from build123d import *

# Parameters (mm, degrees)
SKETCH1_R             = 8
BOSS_EXTRUDE1_DEPTH   = 47.5
BOSS_EXTRUDE2_START   = 15
BOSS_EXTRUDE2_DEPTH   = 10
SKETCH3_R             = 9
BOSS_EXTRUDE3_DEPTH   = 4
LPATTERN1_COUNT       = 6
LPATTERN1_PITCH       = 95
BODY_MOVE_COPY1_ANGLE = 60
BODY_MOVE_COPY2_ANGLE = 120
BODY_MOVE_COPY3_ANGLE = 60
BODY_MOVE_COPY4_ANGLE = 120
BODY_MOVE_COPY5_ANGLE = 180
BOSS_EXTRUDE4_START   = 10
SKETCH4_R             = 8
BOSS_EXTRUDE4_DEPTH   = 10
BOSS_EXTRUDE5_START   = 5
SKETCH5_R             = 9
BOSS_EXTRUDE5_DEPTH   = 5
SKETCH6_R             = 7.5
BOSS_EXTRUDE6_DEPTH   = 5
SKETCH7_R             = 8
BOSS_EXTRUDE7_DEPTH   = 7.5
SKETCH8_R             = 9
BOSS_EXTRUDE8_DEPTH   = 5
BOSS_EXTRUDE9_START   = 23
SKETCH9_R             = 7.5
BOSS_EXTRUDE9_DEPTH   = 23
SKETCH10_R            = 25
SKETCH10_R_2          = 2.5
BOSS_EXTRUDE10_DEPTH  = 10
FILLET1_R             = 2
CUT_EXTRUDE1_REACH    = 638.483
SKETCH11_R            = 2.5


with BuildPart() as part:
    # Sketch1 → Boss-Extrude1 (new, symmetric)
    with BuildSketch(Plane(origin=(0, 0, 0), x_dir=(0, 0, -1), z_dir=(1, 0, 0))):
        Circle(SKETCH1_R)
    extrude(amount=BOSS_EXTRUDE1_DEPTH, both=True)

    # Sketch2 → Boss-Extrude2 (add)
    with BuildSketch(Plane(origin=(0, 0, 0), x_dir=(0, 0, -1), z_dir=(1, 0, 0)).offset(BOSS_EXTRUDE2_START)):
        with BuildLine():
            Line((-3.807936598, -13.756953924), (-8.746197071, -4.848096202))
            ThreePointArc((-8.746197071, -4.848096202), (0, 10), (8.746197071, -4.848096202))
            Line((8.746197071, -4.848096202), (3.807936598, -13.756953924))
            ThreePointArc((3.807936598, -13.756953924), (0, -16), (-3.807936598, -13.756953924))
        make_face()
    boss_extrude2 = extrude(amount=BOSS_EXTRUDE2_DEPTH)

    # Mirror1: Boss-Extrude2 across plane
    add(boss_extrude2.mirror(Plane(origin=(0, 0, 0), x_dir=(0, 0, 1), z_dir=(1, 0, 0))))

    # Sketch3 → Boss-Extrude3 (add, symmetric)
    with BuildSketch(Plane(origin=(0, 0, 0), x_dir=(0, 0, -1), z_dir=(1, 0, 0))):
        Circle(SKETCH3_R)
    extrude(amount=BOSS_EXTRUDE3_DEPTH, both=True)


with BuildPart() as lpattern1_1:
    # LPattern1: pattern copy
    add(part.part.moved(Location(Vector(1, 0, 0) * (1 * LPATTERN1_PITCH))))


with BuildPart() as lpattern1_2:
    # LPattern1: pattern copy
    add(part.part.moved(Location(Vector(1, 0, 0) * (2 * LPATTERN1_PITCH))))


with BuildPart() as lpattern1_3:
    # LPattern1: pattern copy
    add(part.part.moved(Location(Vector(1, 0, 0) * (3 * LPATTERN1_PITCH))))


with BuildPart() as lpattern1_4:
    # LPattern1: pattern copy
    add(part.part.moved(Location(Vector(1, 0, 0) * (4 * LPATTERN1_PITCH))))


with BuildPart() as lpattern1_5:
    # LPattern1: pattern copy
    add(part.part.moved(Location(Vector(1, 0, 0) * (5 * LPATTERN1_PITCH))))


with BuildPart() as lpattern1_3_1:
    # Body-Move_Copy1: moved
    add(lpattern1_3.part.rotate(Axis((0, 0, 0), (-1, 0, 0)), BODY_MOVE_COPY1_ANGLE))


with BuildPart() as lpattern1_1_1:
    # Body-Move_Copy2: moved
    add(lpattern1_1.part.rotate(Axis((0, 0, 0), (-1, 0, 0)), BODY_MOVE_COPY2_ANGLE))


with BuildPart() as lpattern1_4_1:
    # Body-Move_Copy3: moved
    add(lpattern1_4.part.rotate(Axis((0, 0, 0), (1, 0, 0)), BODY_MOVE_COPY3_ANGLE))


with BuildPart() as lpattern1_2_1:
    # Body-Move_Copy4: moved
    add(lpattern1_2.part.rotate(Axis((0, 0, 0), (1, 0, 0)), BODY_MOVE_COPY4_ANGLE))


with BuildPart() as lpattern1_5_1:
    # Body-Move_Copy5: moved
    add(lpattern1_5.part.rotate(Axis((0, 0, 0), (1, 0, 0)), BODY_MOVE_COPY5_ANGLE))

    # Sketch4 → Boss-Extrude4 (add)
    with BuildSketch(Plane(origin=(522.5, 0, 0), x_dir=(0, 0, -1), z_dir=(1, 0, 0)).offset(BOSS_EXTRUDE4_START)):
        with Locations(Location((0, 0, 0), (0, 0, 180))):
            Circle(SKETCH4_R)
    extrude(amount=-BOSS_EXTRUDE4_DEPTH)

    # Sketch5 → Boss-Extrude5 (add)
    with BuildSketch(Plane(origin=(532.5, 0, 0), x_dir=(0, 0, -1), z_dir=(1, 0, 0)).offset(BOSS_EXTRUDE5_START)):
        with Locations(Location((0, 0, 0), (0, 0, 180))):
            Circle(SKETCH5_R)
    extrude(amount=-BOSS_EXTRUDE5_DEPTH)


with BuildPart() as part_1:
    add(part.part)

    # Combine1: union LPattern1_1, LPattern1_2, LPattern1_3, LPattern1_4, LPattern1_5
    add(lpattern1_1_1.part)
    add(lpattern1_2_1.part)
    add(lpattern1_3_1.part)
    add(lpattern1_4_1.part)
    add(lpattern1_5_1.part)

    # Sketch6 → Boss-Extrude6 (add)
    with BuildSketch(Plane(origin=(537.5, 0, 0), x_dir=(0, 0, -1), z_dir=(1, 0, 0))):
        Circle(SKETCH6_R)
    extrude(amount=BOSS_EXTRUDE6_DEPTH)

    # Sketch7 → Boss-Extrude7 (add)
    with BuildSketch(Plane.ZY.offset(47.5)):
        with Locations(Location((0, 0, 0), (0, 0, 180))):
            Circle(SKETCH7_R)
    extrude(amount=BOSS_EXTRUDE7_DEPTH)

    # Sketch8 → Boss-Extrude8 (add)
    with BuildSketch(Plane.ZY.offset(55)):
        with Locations(Location((0, 0, 0), (0, 0, 180))):
            Circle(SKETCH8_R)
    extrude(amount=BOSS_EXTRUDE8_DEPTH)

    # Sketch9 → Boss-Extrude9 (add)
    with BuildSketch(Plane.ZY.offset(60).offset(BOSS_EXTRUDE9_START)):
        with Locations(Location((0, 0, 0), (0, 0, 180))):
            Circle(SKETCH9_R)
    extrude(amount=-BOSS_EXTRUDE9_DEPTH)

    # Sketch10 → Boss-Extrude10 (add)
    with BuildSketch(Plane.ZY.offset(83)):
        Circle(SKETCH10_R)
        Circle(SKETCH10_R_2, mode=Mode.SUBTRACT)
    extrude(amount=BOSS_EXTRUDE10_DEPTH)

    # Fillet1
    fillet1_edges = [part_1.edges().sort_by_distance(p)[0] for p in [
        (-83, 0, 7.5),
        (-83, 0, -25),
    ]]
    fillet(fillet1_edges, radius=FILLET1_R)

    # Sketch11 → Cut-Extrude1 (cut, up to next)
    with BuildSketch(Plane.ZY.offset(93), mode=Mode.PRIVATE) as cut_extrude1_sk1:
        with Locations((0, 15)):
            Circle(SKETCH11_R)
    cut_extrude1_tool1 = extrude(cut_extrude1_sk1.sketch, amount=-CUT_EXTRUDE1_REACH, mode=Mode.PRIVATE) & part_1.part
    # Sketch11 → Cut-Extrude1 (cut, up to next)
    with BuildSketch(Plane.ZY.offset(93), mode=Mode.PRIVATE) as cut_extrude1_sk2:
        with Locations((14.265847744, 4.635254916)):
            Circle(SKETCH11_R)
    cut_extrude1_tool2 = extrude(cut_extrude1_sk2.sketch, amount=-CUT_EXTRUDE1_REACH, mode=Mode.PRIVATE) & part_1.part
    # Sketch11 → Cut-Extrude1 (cut, up to next)
    with BuildSketch(Plane.ZY.offset(93), mode=Mode.PRIVATE) as cut_extrude1_sk3:
        with Locations((8.816778784, -12.135254916)):
            Circle(SKETCH11_R)
    cut_extrude1_tool3 = extrude(cut_extrude1_sk3.sketch, amount=-CUT_EXTRUDE1_REACH, mode=Mode.PRIVATE) & part_1.part
    # Sketch11 → Cut-Extrude1 (cut, up to next)
    with BuildSketch(Plane.ZY.offset(93), mode=Mode.PRIVATE) as cut_extrude1_sk4:
        with Locations((-8.816778784, -12.135254916)):
            Circle(SKETCH11_R)
    cut_extrude1_tool4 = extrude(cut_extrude1_sk4.sketch, amount=-CUT_EXTRUDE1_REACH, mode=Mode.PRIVATE) & part_1.part
    # Sketch11 → Cut-Extrude1 (cut, up to next)
    with BuildSketch(Plane.ZY.offset(93), mode=Mode.PRIVATE) as cut_extrude1_sk5:
        with Locations((-14.265847744, 4.635254916)):
            Circle(SKETCH11_R)
    cut_extrude1_tool5 = extrude(cut_extrude1_sk5.sketch, amount=-CUT_EXTRUDE1_REACH, mode=Mode.PRIVATE) & part_1.part
    add(cut_extrude1_tool1.solids().sort_by_distance((-93, 15, 0))[0], mode=Mode.SUBTRACT)
    add(cut_extrude1_tool2.solids().sort_by_distance((-93, 4.635255, 14.265848))[0], mode=Mode.SUBTRACT)
    add(cut_extrude1_tool3.solids().sort_by_distance((-93, -12.135255, 8.816779))[0], mode=Mode.SUBTRACT)
    add(cut_extrude1_tool4.solids().sort_by_distance((-93, -12.135255, -8.816779))[0], mode=Mode.SUBTRACT)
    add(cut_extrude1_tool5.solids().sort_by_distance((-93, 4.635255, -14.265848))[0], mode=Mode.SUBTRACT)


solid = part_1.part
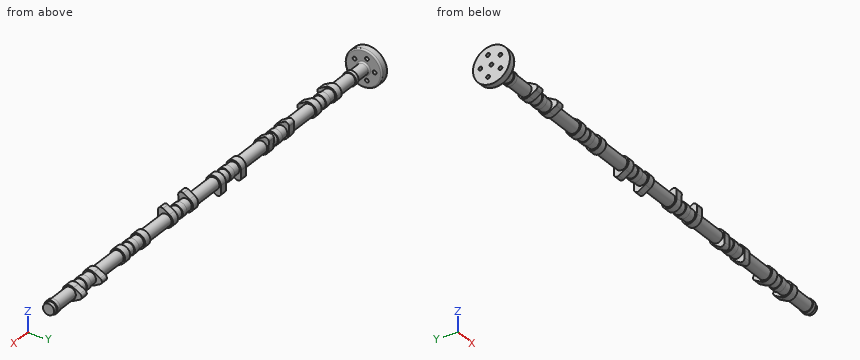
Work out the finished part from the listing and answer in its coordinate system (mm). Round coordinates to 2 decimals unless told otherwise and drop trailing zeros. Write each loop counter-clockwise with the first axis right and the second up, starting at its lowest first coordinate (ties: lowest second). Pieces come first, ordered by that corner, then holes. Notation, with made-up numbers: (0.5, 14) -> (9.5, 14) arc R19 cw to (9.5, 51) -> close; hole circle Ø3 at (-33, 13.25). An arc over 180 degrees is marked (long way). Answer as CSV lines item,"result". Start each with the question number.
(1) The part is cut by section A-A, the plane x = 152. Give the vertices of the cut face in (y, z).
(2) Each of these flat-tipped pins is pushed along its axis until it touches: pin 1 (8 mm diameter, centred on y = 15, z = 0, fed in from +X); pin 2 (12 mm diameter, centred on x = 121.5, z = -13, fed in from -Y); pin 3 (5 mm diameter, centred on x = 98, z = 8, fed in from -Y). Where does it stop, or does it pass through?
(3) Find the intervals of material crossed by probe 1 along X at (y, z) = (4, -11); probe 2 along X at (y, z) = (-11, 0); probe 3 along Y at (x, z) = (-85, 0), in increasing order.
Output values:
1,outline,"circle Ø16 at (0, 0)"
2,pin 1,"stops at x = 500"
2,pin 2,"stops at y = -6.95"
2,pin 3,"stops at y = -7.12"
3,probe 1,"x = -93 to -83, 165 to 175, 205 to 215"
3,probe 2,"x = -93 to -83, -25 to -15, 15 to 25"
3,probe 3,"y = -25 to -2.5, 2.5 to 12.5, 17.5 to 25"
